Could you check a few things on this model? Use its own coordinates, in mm. Face numbers are marked on the shaded views. A direction names the side the tool comes from. Give positions to 0.01 mm unless a question says otherwise; leave off trailing zeros. Write each loop counter-clockwise with the first axis right and the second up, starting at its lowest first coordinate (ties: lowest second). Pieces come first, ordered by that corner, then holes. Notation, with made-up numbers: (60.25, 53) - (116.25, 53) arc R12 cw to (116.25, 72) - close; hole circle Ø2 at (-22, 47). An arc over 180 degrees is marked (long way). Answer in a Markdown table with one row per item.
from build123d import *

# Parameters (mm, degrees)
BOSS_EXTRUDE1_DEPTH = 15
SKETCH3_R           = 2
CUT_EXTRUDE2_DEPTH  = 2.5
SKETCH4_R           = 1
CUT_EXTRUDE3_DEPTH  = 3
SKETCH2_W           = 4
SKETCH2_H           = 4.5
CUT_EXTRUDE1_DEPTH  = 6
SKETCH5_W           = 1.2
SKETCH5_H           = 2
CUT_EXTRUDE4_DEPTH  = 5.2
SKETCH6_W           = 0.5
SKETCH6_H           = 6
BOSS_EXTRUDE2_DEPTH = 0.5
SKETCH7_W           = 0.5
SKETCH7_H           = 6
CUT_EXTRUDE5_DEPTH  = 0.5
LPATTERN1_COUNT     = 3
LPATTERN1_PITCH     = 5
CUT_EXTRUDE6_DEPTH  = 10
BOSS_EXTRUDE3_DEPTH = 6


with BuildPart() as part:
    # Sketch1 → Boss-Extrude1 (new body)
    with BuildSketch(Plane.XY):
        Polygon((2.7, 5.1), (-2.7, 5.1), (-2.7, 1.4), (-3.9, 1.4), (-3.9, -5.1), (3.9, -5.1), (3.9, 1.4), align=None)
    extrude(amount=-BOSS_EXTRUDE1_DEPTH)

    # Sketch3 → Cut-Extrude2 (cut)
    with BuildSketch(Plane(origin=(0, 5.1, 0), x_dir=(1, 0, 0), z_dir=(0, 1, 0))):
        with Locations((0, 2.5)):
            Circle(SKETCH3_R)
        with Locations((0, 7.5)):
            Circle(SKETCH3_R)
        with Locations((0, 12.5)):
            Circle(SKETCH3_R)
    extrude(amount=-CUT_EXTRUDE2_DEPTH, mode=Mode.SUBTRACT)

    # Sketch4 → Cut-Extrude3 (cut)
    with BuildSketch(Plane(origin=(0, 2.6, 0), x_dir=(1, 0, 0), z_dir=(0, 1, 0))):
        with Locations((0, 2.5)):
            Circle(SKETCH4_R)
        with Locations((0, 7.5)):
            Circle(SKETCH4_R)
        with Locations((0, 12.5)):
            Circle(SKETCH4_R)
    extrude(amount=-CUT_EXTRUDE3_DEPTH, mode=Mode.SUBTRACT)

    # Sketch2 → Cut-Extrude1 (cut)
    with BuildSketch(Plane(origin=(3.9, 0, 0), x_dir=(0, 0, -1), z_dir=(1, 0, 0))):
        with Locations((2.5, -1.85)):
            Rectangle(SKETCH2_W, SKETCH2_H)
    cut_extrude1 = extrude(amount=-CUT_EXTRUDE1_DEPTH, mode=Mode.SUBTRACT)

    # Sketch5 → Cut-Extrude4 (cut)
    with BuildSketch(Plane(origin=(3.9, 0, 0), x_dir=(0, 0, -1), z_dir=(1, 0, 0))):
        with Locations((2.5, -5.1)):
            Rectangle(SKETCH5_W, SKETCH5_H)
    cut_extrude4 = extrude(amount=-CUT_EXTRUDE4_DEPTH, mode=Mode.SUBTRACT)

    # Sketch6 → Boss-Extrude2 (add)
    with BuildSketch(Plane.XY):
        with Locations((-2.75, -2.1)):
            Rectangle(SKETCH6_W, SKETCH6_H)
    extrude(amount=BOSS_EXTRUDE2_DEPTH)

    # Sketch7 → Cut-Extrude5 (cut)
    with BuildSketch(Plane(origin=(0, 0, -15), x_dir=(-1, 0, 0), z_dir=(0, 0, -1))):
        with Locations((2.75, -2.1)):
            Rectangle(SKETCH7_W, SKETCH7_H)
    extrude(amount=-CUT_EXTRUDE5_DEPTH, mode=Mode.SUBTRACT)

    # LPattern1: Cut-Extrude1, Cut-Extrude4 ×3
    with Locations(*[(0, 0, -i * LPATTERN1_PITCH) for i in range(1, LPATTERN1_COUNT)]):
        add(cut_extrude1, mode=Mode.SUBTRACT)
        add(cut_extrude4, mode=Mode.SUBTRACT)

    # Sketch8 → Cut-Extrude6 (cut)
    with BuildSketch(Plane(origin=(0, 0.9, 0), x_dir=(1, 0, 0), z_dir=(0, 1, 0))):
        Polygon((-3, -0.5), (-2.89, 0), (-3, 0), align=None)
        Polygon((-2.5, -0.5), (-2.61, 0), (-2.5, 0), align=None)
    extrude(amount=-CUT_EXTRUDE6_DEPTH, mode=Mode.SUBTRACT)

    # Sketch9 → Boss-Extrude3 (add)
    with BuildSketch(Plane.XZ.offset(5.1)):
        Polygon((-3, -14.5), (-2.89, -15), (-3, -15), align=None)
        Polygon((-2.5, -14.5), (-2.61, -15), (-2.5, -15), align=None)
    extrude(amount=-BOSS_EXTRUDE3_DEPTH)


solid = part.part
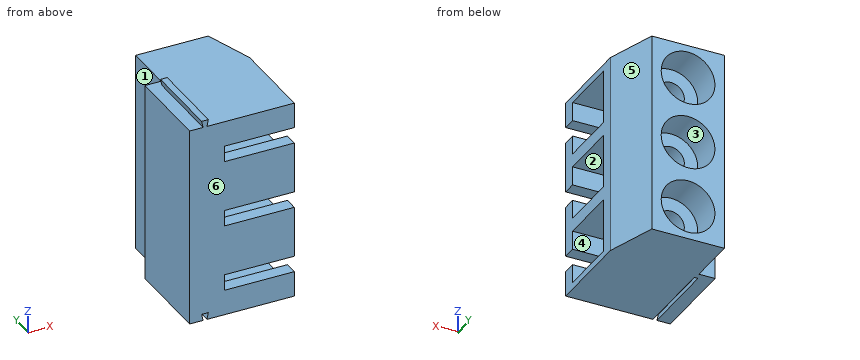
1) We'd pull the mould along Y, two halves only. Please class the marked faces 4, 5 and 6: +Y half, -Y half, draft (parallel to the pull), parting line (faces both ways), or undercut.
Check values:
| item | result |
|---|---|
| face 4 | undercut |
| face 5 | +Y half |
| face 6 | -Y half |
2) Imagine slicing it at B-B (y = -3). List the corners of the cut face in (x, z) for me, then the cut area to 3 significant figures.
Check values:
| item | result |
|---|---|
| outline | (-3.9, -15) - (-2.89, -15) - (-3, -14.5) - (-2.5, -14.5) - (-2.61, -15) - (3.9, -15) - (3.9, -14.5) - (-2.1, -14.5) - (-2.1, -10.5) - (3.9, -10.5) - (3.9, -9.5) - (-2.1, -9.5) - (-2.1, -5.5) - (3.9, -5.5) - (3.9, -4.5) - (-2.1, -4.5) - (-2.1, -0.5) - (3.9, -0.5) - (3.9, 0) - (-2.61, 0) - (-2.5, 0.5) - (-3, 0.5) - (-2.89, 0) - (-3.9, 0) - close |
| area | 45.0 mm2 |
3) Imagine slicing it at A-A (z = -12.5). List the corners of the cut face in (x, y) for me, then the cut area to 3 significant figures.
Check values:
| item | result |
|---|---|
| outline | (-3.9, -5.1) - (-1.3, -5.1) - (-1.3, -4.1) - (-2.1, -4.1) - (-2.1, 0.4) - (-1, 0.4) - (-1, 2.6) - (-2, 2.6) - (-2, 5.1) - (-2.7, 5.1) - (-2.7, 1.4) - (-3.9, 1.4) - close; (1, 0.4) - (3.9, 0.4) - (3.9, 1.4) - (2.7, 5.1) - (2, 5.1) - (2, 2.6) - (1, 2.6) - close |
| area | 26.3 mm2 |
4) Imagine slicing it at D-D (x = 0). State how many separate pieces and enclosed holes the cut face has, then the cut area to 3 significant figures.
Check values:
| item | result |
|---|---|
| separate pieces | 4 |
| enclosed holes | 0 |
| area | 52.2 mm2 |
5) Will these pins go through, and if not, where does the flat tip stop? P1, Ø0.5, axis at y = -5, z = -7.5, coming from the +X side; P2, Ø0.8, axis at x = 0.5, y = -4.5, coming from the +Z side.
Check values:
| item | result |
|---|---|
| P1 | stops at x = -1.3 |
| P2 | stops at z = 0 |
6) If I drill on line 1 (Z direction, x = 0.5, y = 0); line 2 (Z direction, x = 0.25, y = -4.25); line 3 (Y direction, x = 2.25, z = -4), over which ranges is the centre line in solid material (lowest first)?
Check values:
| item | result |
|---|---|
| line 1 | z = -15 to -14.5, -10.5 to -9.5, -5.5 to -4.5, -0.5 to 0 |
| line 2 | z = -15 to -13.1, -11.9 to -8.1, -6.9 to -3.1, -1.9 to 0 |
| line 3 | y = -5.1 to -4.1, 0.4 to 5.1 |
7) Imagine slicing it at C-C (z = -4.75). List the corners of the cut face in (x, y) for me.
Check values:
| item | result |
|---|---|
| outline | (-3.9, -5.1) - (3.9, -5.1) - (3.9, 1.4) - (2.7, 5.1) - (-2.7, 5.1) - (-2.7, 1.4) - (-3.9, 1.4) - close |
8) On a 3-axis mill with a long thin cutter (end or side, diameter ignored), from which of +Z, -Z, +X, -X, +Y, -Y can I reach the whole of each face in a straight line? I mean the marked faces 1, 2 and 3. Say none if no direction works.
Check values:
| item | result |
|---|---|
| face 1 | +Z, -Z, -X, +Y |
| face 2 | +X |
| face 3 | +Y |
